Geometry check sheet. Reference: the model listing, model coordinates, mm. A direction names the side the tool comes from. Coordinates: 2 decimals unless noted, no trailing zeros. Order: outer loops, then holes, each group sorted by start corner. A loop starts at its lowest first (then second) coordinate and runs counter-clockwise, first axis right, second up. Notation, with made-up numbers: M -23.75,-23 L 30.25,-23 A14 ccw 30.25,4 Z; hole C 28.5,54 d1. An arc over 180 degrees is marked long. Use CSV: the item, a comma, the result in double quotes. Start each with the question number.
```python
from build123d import *

# Parameters (mm, degrees)
SKETCH1_W           = 100
SKETCH1_H           = 50
SKETCH1_R           = 2.5
SKETCH1_W_2         = 5
SKETCH1_H_2         = 40
BOSS_EXTRUDE1_DEPTH = 8


with BuildPart() as part:
    # Sketch1 → Boss-Extrude1 (new body)
    with BuildSketch(Plane.XY):
        Rectangle(SKETCH1_W, SKETCH1_H)
        with Locations((-13, -16.244168493)):
            Circle(SKETCH1_R, mode=Mode.SUBTRACT)
        with Locations((13, -16.244168493)):
            Circle(SKETCH1_R, mode=Mode.SUBTRACT)
        with Locations((-37.5, 0)):
            Rectangle(SKETCH1_W_2, SKETCH1_H_2, mode=Mode.SUBTRACT)
        with Locations((37.5, 0)):
            Rectangle(SKETCH1_W_2, SKETCH1_H_2, mode=Mode.SUBTRACT)
    extrude(amount=BOSS_EXTRUDE1_DEPTH)


solid = part.part
```
1) Gauge pin test, flat end, axial feed: P1, Ø6.5, axis at x = 13, y = -16.24, coming from the +Z side. Record the tip position at first contact, or that the pin passes through.
2) Section check D-D on y = -17.5. Record the boundary of the cut face in (x, z).
3) Draft check along Y on faces 3 (the face through (50, 0, 4)), 4 (the face through (-1, 25, 4)), 5 (the face through (11.02, -17.77, 3.94)). Enter one of: +Y half, -Y half, draft (parallel to the pull), parting line (faces both ways), or undercut.
4) Material ranges on line 1 along X through (y, z) = (4, 4); line 2 along Y through (x, z) = (-13, 3); line 3 along Y through (x, z) = (11, 2.5), recorded low to high.
5) Section check C-C on x = 13. Record the boundary of the cut face in (y, z), then the cut area to 3 significant figures.
6) Section check A-A on y = 19. Record the boundary of the cut face in (x, z), then the cut area to 3 significant figures.
7) Set-up check for faces 1 (the face through (-1, -25, 4)), 2 (the face through (37, -20, 4)): record each of +Z, -Z, +X, -X, +Y, -Y from which the full face is reachable in a straight line by a thin tool's end or side.
8) Section check B-B on x = -38. Record the boundary of the cut face in (y, z), then the cut area to 3 significant figures.
Results are:
1,P1,"stops at z = 8"
2,outline,"M -50,0 L -40,0 L -40,8 L -50,8 Z; M -35,0 L -15.16,0 L -15.16,8 L -35,8 Z; M -10.84,0 L 10.84,0 L 10.84,8 L -10.84,8 Z; M 15.16,0 L 35,0 L 35,8 L 15.16,8 Z; M 40,0 L 50,0 L 50,8 L 40,8 Z"
3,face 3,"draft"
3,face 4,"+Y half"
3,face 5,"undercut"
4,line 1,"x = -50 to -40, -35 to 35, 40 to 50"
4,line 2,"y = -25 to -18.74, -13.74 to 25"
4,line 3,"y = -25 to -17.74, -14.74 to 25"
5,outline,"M -25,0 L -18.74,0 L -18.74,8 L -25,8 Z; M -13.74,0 L 25,0 L 25,8 L -13.74,8 Z"
5,area,"360 mm²"
6,outline,"M -50,0 L -40,0 L -40,8 L -50,8 Z; M -35,0 L 35,0 L 35,8 L -35,8 Z; M 40,0 L 50,0 L 50,8 L 40,8 Z"
6,area,"720 mm²"
7,face 1,"+Z, -Z, +X, -X, -Y"
7,face 2,"+Z, -Z"
8,outline,"M -25,0 L -20,0 L -20,8 L -25,8 Z; M 20,0 L 25,0 L 25,8 L 20,8 Z"
8,area,"80.0 mm²"
